from build123d import *

# Parameters (mm, degrees)
SKETCH1_W           = 76
SKETCH1_H           = 40.5
BOSS_EXTRUDE1_DEPTH = 9
SHELL1_T            = -1.5
SKETCH2_W           = 1.5
SKETCH2_H           = 73
BOSS_EXTRUDE2_DEPTH = 16.5
SKETCH3_R           = 0.6
BOSS_EXTRUDE3_DEPTH = 5


with BuildPart() as part:
    # Sketch1 → Boss-Extrude1 (new, symmetric)
    with BuildSketch(Plane(origin=(0, 0, 0), x_dir=(0, 1, 0), z_dir=(0, 0, 1))):
        Rectangle(SKETCH1_W, SKETCH1_H)
    extrude(amount=BOSS_EXTRUDE1_DEPTH, both=True)

    # Shell1
    shell1_openings = [part.faces().sort_by_distance(p)[0] for p in [
        (0, 0, 9),
    ]]
    offset(amount=SHELL1_T, openings=shell1_openings, kind=Kind.INTERSECTION)

    # Sketch2 → Boss-Extrude2 (add)
    with BuildSketch(Plane.XY.offset(-7.5)):
        Rectangle(SKETCH2_W, SKETCH2_H)
    extrude(amount=BOSS_EXTRUDE2_DEPTH)

    # Sketch3 → Boss-Extrude3 (add)
    with BuildSketch(Plane(origin=(0, 38, 0), x_dir=(-1, 0, 0), z_dir=(0, 1, 0))):
        with Locations(Location((3, -7, 0), (0, 0, 270))):
            Circle(SKETCH3_R)
        with Locations(Location((-3, -7, 0), (0, 0, 270))):
            Circle(SKETCH3_R)
    extrude(amount=BOSS_EXTRUDE3_DEPTH)


solid = part.part
Geometry check sheet. Reference: the model listing, model coordinates, mm. A direction names the side the tool comes from. Give positions to 0.01 mm unless a question says otherwise; leave off trailing zeros. Loops run counter-clockwise (first coordinate to the right, second up) from the corner with the lowest first, then second, coordinate; pieces in that order, holes last. Notation, with made-up numbers: M 33,58 L 70,58 A19 cw 70,76 Z; hole C 70,35 d11. An arc over 180 degrees is marked long. Answer as a JSON object with one key per item and string values. Group by question number.
Item 1: Mould release check, pull along X, two halves, no side actions. Record for faces 3 (the flat face through (0, -1, -9)), 4 (the flat face through (-20.25, -1, 0)), 5 (the flat face through (10, 36.5, 1)): pulls with the +X half, pulls with the -X half, needs draft (parallel to the pull), parting line crosses it, or undercut.
Item 2: Sectioned sample at B-B on x = 11.5. Record the boundary of the cut face in (y, z), plus the area to 4 significant figures.
Item 3: Gauge pin test, flat ends, axial feed: pin 1 (4 mm diameter, centred on x = -15.5, z = -7, fed in from +Y); pin 2 (9 mm diameter, centred on x = -13, y = 8.5, fed in from +Z). Record the tip position at first contact, or that the pin passes through.
Item 4: Sectioned sample at A-A on y = -5.5. Record the boundary of the cut face in (x, z).
Item 5: Material ranges on L1, parallel to X at y = -11, z = 1.25; L2, parallel to Y at x = -5, z = -6.5; L3, parallel to Z at x = 5.5, y = 16, recorded low to high.
Item 6: Access from +Z, -Z, +X, -X, +Y, -Y to the whole of each face (thin tool, end or side, straight path). Record for faces 1 (the flat face through (0.75, -1, 1)), 2 (the flat face through (0, -11, 9)).
Item 7: Sectioned sample at C-C on z = 1.5. Record the boundary of the cut face in (x, y).
Findings below:
{
 "1": {"face 3": "needs draft", "face 4": "pulls with the -X half", "face 5": "undercut"},
 "2": {"outline": "M -38,-9 L 38,-9 L 38,9 L 36.5,9 L 36.5,-7.5 L -36.5,-7.5 L -36.5,9 L -38,9 Z", "area": "163.5 mm2"},
 "3": {"pin 1": "y = 38", "pin 2": "z = -7.5"},
 "4": {"outline": "M -20.25,-9 L 20.25,-9 L 20.25,9 L 18.75,9 L 18.75,-7.5 L 0.75,-7.5 L 0.75,9 L -0.75,9 L -0.75,-7.5 L -18.75,-7.5 L -18.75,9 L -20.25,9 Z"},
 "5": {"L1": "-20.25 to -18.75, -0.75 to 0.75, 18.75 to 20.25", "L2": "-38 to -36.5, 36.5 to 38", "L3": "-9 to -7.5"},
 "6": {"face 1": "+Z", "face 2": "+Z, +X, -X, +Y, -Y"},
 "7": {"outline": "M -20.25,-38 L 20.25,-38 L 20.25,38 L -20.25,38 Z; hole M -18.75,-36.5 L -0.75,-36.5 L -0.75,36.5 L -18.75,36.5 Z; hole M 0.75,-36.5 L 18.75,-36.5 L 18.75,36.5 L 0.75,36.5 Z"}
}
